Design review of the part built by this model. Coordinates are the model's own, in mm. Face numbers are marked on the shaded views. Coordinates: 2 decimals unless noted, no trailing zeros. Write each loop counter-clockwise with the first axis right and the second up, starting at its lowest first coordinate (ties: lowest second). Pieces come first, ordered by that corner, then holes. Notation, with made-up numbers: (20, -9.75) -> (49, -9.75) arc R23 cw to (49, 10.25) -> close; hole circle Ø11 at (78.25, -19.5). An arc over 180 degrees is marked (long way). Return JSON: item names as keys, results as strings. Group by question number.
Autodesk Inventor part; units mm, degrees
ref_plane "YZ Plane" through (0, 0, 0) normal (1, 0, 0) x (0, 1, 0)
ref_plane "XZ Plane" through (0, 0, 0) normal (0, 1, 0) x (-1, 0, 0)
ref_plane "XY Plane" through (0, 0, 0) normal (0, 0, 1) x (1, 0, 0)
sketch "Sketch1" plane through (0, 0, 0) normal (0, 1, 0) x (-1, 0, 0)
  line L0 (-34.1, -49) -> (34.1, -49)
  line L1 (34.1, -49) -> (34.1, 49)
  line L2 (34.1, 49) -> (-34.1, 49)
  line L3 (-34.1, 49) -> (-34.1, -49)
  line L4 (-34.1, -49) -> (34.1, 49) construction
  line L5 (34.1, -49) -> (-34.1, 49) construction
  circle A0 centre (-16.9, 39.55) radius 2
  circle A1 centre (-16.9, 39.55) radius 3.25
  line L6 (-18.8909, 27.1453) -> (-18.8909, 26.9568)
  circle A2 centre (-10.1, -20) radius 2
  circle A3 centre (-10.1, -20) radius 3.25
  point P0 (0, 0)
  dimension "d0" = 68.2
  dimension "d1" = 98
  dimension "d6" = 4
  dimension "d7" = 6.5
  dimension "d8" = 17.2
  dimension "d9" = 9.45
  dimension "d10" = 24
  dimension "d11" = 29
  dimension "d12" = 4
  dimension "d13" = 6.5
extrude "Extrusion1" add sketch "Sketch1" along normal blind 31.8 contours L3 L2 L1 L0 | A0 | A1 | A2 | A3
shell "Shell1" thickness 1.5 removed faces 1 at (11.3667, 31.8, 16.3333)
extrude "Extrusion2" add sketch "Sketch1" along normal blind 4.5 contours A1 | A3
sketch "Sketch2" plane through (-34.1, 0, 49) normal (0, 0, 1) x (1, 0, 0)
  line L0 (0, 0) -> (68.2, 0)
  line L1 (68.2, 0) -> (68.2, 31.8)
  line L2 (68.2, 0) -> (68.2, 31.8)
  line L3 (68.2, 1.5) -> (40, 1.5)
  line L4 (68, 6) -> (36, 6)
  line L5 (36, 6) -> (36, 4.5)
  line L6 (36, 4.5) -> (68, 4.5)
  line L7 (68, 4.5) -> (68, 6)
  line L8 (47.2, 17.65) -> (54.7, 17.65)
  line L9 (54.7, 17.65) -> (54.7, 14.9)
  line L10 (54.7, 14.9) -> (47.2, 14.9)
  line L11 (47.2, 14.9) -> (47.2, 17.65)
  line L12 (47.2, 17.65) -> (54.7, 14.9)
  line L13 (54.7, 17.65) -> (47.2, 14.9)
  line L14 (55.7, 13.9) -> (46.2, 13.9)
  line L15 (46.2, 13.9) -> (46.2, 18.65)
  line L16 (46.2, 18.65) -> (55.7, 18.65)
  line L17 (55.7, 18.65) -> (55.7, 13.9)
  line L18 (55.7, 13.9) -> (46.2, 18.65) construction
  line L19 (46.2, 13.9) -> (55.7, 18.65) construction
  point P0 (34.1, 0)
  point P1 (50.95, 16.275)
  dimension "d19" = 1.5
  dimension "d20" = 3
  dimension "d21" = 1.5
  dimension "d22" = 8.9
  dimension "d23" = 7.5
  dimension "d24" = 2.75
  dimension "d25" = 13.5
  dimension "d26" = 1
  dimension "d27" = 1
extrude "Extrusion3" cut sketch "Sketch2" against normal blind 4.5 contours L12 L13 L11 | L8 L13 L12 | L9 L12 L13 | L13 L12 L10 | L14 L15 L16 L17
fillet "Fillet1" radius 1 4 edges at (16.85, 18.65, 49) (21.6, 16.275, 49) (16.85, 13.9, 49) (12.1, 16.275, 49)
sketch "Sketch3" plane through (34.1, 0, 49) normal (1, 0, 0) x (0, 0, -1)
  line L0 (0, 0) -> (98, 0)
  line L1 (98, 0) -> (98, 31.8)
  line L2 (80.7, 17.4) -> (93.6, 17.4)
  line L3 (93.6, 17.4) -> (93.6, 6)
  line L4 (93.6, 6) -> (80.7, 6)
  line L5 (80.7, 6) -> (80.7, 17.4)
  line L6 (80.7, 17.4) -> (93.6, 6) construction
  line L7 (93.6, 17.4) -> (80.7, 6) construction
  line L8 (94.6, 5) -> (79.7, 5)
  line L9 (79.7, 5) -> (79.7, 18.4)
  line L10 (79.7, 18.4) -> (94.6, 18.4)
  line L11 (94.6, 18.4) -> (94.6, 5)
  line L12 (94.6, 5) -> (79.7, 18.4) construction
  line L13 (79.7, 5) -> (94.6, 18.4) construction
  point P0 (49, 0)
  point P1 (87.15, 11.7)
  point P2 (87.15, 11.7)
  dimension "d31" = 6
  dimension "d32" = 4.4
  dimension "d33" = 11.4
  dimension "d34" = 12.9
  dimension "d35" = 1
  dimension "d36" = 1
extrude "Extrusion4" cut sketch "Sketch3" against normal blind 4.5 contours L2 L3 L4 L5 | L8 L9 L10 L11
sketch "Sketch4" plane through (34.1, 0, -49) normal (0, 0, -1) x (-1, 0, 0)
  line L0 (0, 0) -> (68.2, 0)
  line L1 (0, 0) -> (0, 31.8)
  line L2 (28.8, 6) -> (20.1, 6)
  line L3 (20.1, 6) -> (20.1, 16.6)
  line L4 (20.1, 16.6) -> (28.8, 16.6)
  line L5 (28.8, 16.6) -> (28.8, 6)
  line L6 (28.8, 6) -> (20.1, 16.6) construction
  line L7 (20.1, 6) -> (28.8, 16.6) construction
  line L8 (29.8, 5) -> (19.1, 5)
  line L9 (19.1, 5) -> (19.1, 17.6)
  line L10 (19.1, 17.6) -> (29.8, 17.6)
  line L11 (29.8, 17.6) -> (29.8, 5)
  line L12 (29.8, 5) -> (19.1, 17.6) construction
  line L13 (19.1, 5) -> (29.8, 17.6) construction
  point P0 (34.1, 0)
  point P1 (24.45, 11.3)
  dimension "d39" = 20.1
  dimension "d40" = 6
  dimension "d41" = 8.7
  dimension "d42" = 10.6
  dimension "d43" = 1
  dimension "d44" = 1
extrude "Extrusion5" cut sketch "Sketch4" against normal blind 4.5 contours L2 L3 L4 L5 | L8 L9 L10 L11
sketch "Sketch5" plane through (0, 31.8, 0) normal (0, 1, 0) x (1, 0, 0)
  line L0 (32.6, -47.5) -> (-32.6, -47.5)
  line L1 (-32.6, -47.5) -> (-32.6, 47.5)
  line L2 (-32.6, 47.5) -> (32.6, 47.5)
  line L3 (32.6, 47.5) -> (32.6, -47.5)
  line L4 (34.1, -49) -> (34.1, 49)
  line L5 (34.1, 49) -> (-34.1, 49)
  line L6 (-34.1, 49) -> (-34.1, -49)
  line L7 (-34.1, -49) -> (34.1, -49)
  line L8 (34.1, -49) -> (-34.1, -49)
  line L9 (-34.1, -49) -> (-34.1, 49)
  line L10 (-34.1, 49) -> (34.1, 49)
  line L11 (34.1, 49) -> (34.1, -49)
  circle A0 centre (-23.6, -34.15) radius 3
  circle A1 centre (-23.6, -34.15) radius 3.5
  circle A2 centre (-5.6, -34.15) radius 3.5
  circle A3 centre (-23.6, -16.15) radius 3.5
  circle A4 centre (-5.6, -16.15) radius 3.5
  circle A5 centre (-23.6, 1.85) radius 3.5
  circle A6 centre (-5.6, 1.85) radius 3.5
  circle A7 centre (-23.6, 19.85) radius 3.5
  circle A8 centre (-5.6, 19.85) radius 3.5
  circle A9 centre (-23.6, 37.85) radius 3.5
  circle A10 centre (-5.6, 37.85) radius 3.5
  circle A11 centre (-5.6, 1.85) radius 3.5
  circle A12 centre (21.9, 19.85) radius 3.5
  circle A13 centre (21.9, 1.85) radius 3.5
  line L12 (34.1, -49) -> (-34.1, -49)
  line L13 (-34.1, -49) -> (-34.1, 49)
  line L14 (-34.1, 49) -> (34.1, 49)
  line L15 (34.1, 49) -> (34.1, -49)
  point P0 (0, 0)
  dimension "d47" = 6
  dimension "d48" = 7
  dimension "d50" = 13.35
  dimension "d51" = 9
  dimension "d54" = 18
  dimension "d57" = 18
  dimension "d62" = 18
  dimension "d65" = 18
  dimension "d70" = 18
  dimension "d73" = 27.5
extrude "Extrusion6" add sketch "Sketch5" along normal blind 1.5 contours L0 L1 L2 L3 | L7 L6 L5 L4
fillet "Fillet2" radius 2 4 edges at (34.1, 16.65, -49) (-34.1, 16.65, -49) (34.1, 16.65, 49) (-34.1, 16.65, 49)
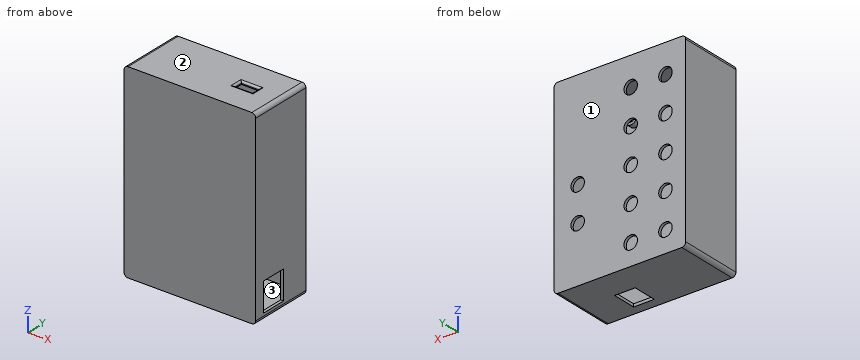
Q1. The part is to be moulded in two halves that separate along Y. For the marked faces 1, 2 and 3, say which applies: +Y half, -Y half, draft (parallel to the pull), parting line (faces both ways), or undercut.
Q2. We need section A-A on y = 30.5. Write out the cut boundary in (x, z).
Q3. Wall thickness on L1, parallel to Z at x = -23.6, y = 32.25; L2, parallel to X at y = 2.1, z = -20; L3, parallel to X at y = 24, z = -3.5: over which ranges is each line inside the solid? List them lowest first.
Q4. We need section C-C on z = 34.15. Write out the cut boundary in (x, y).
Q5. We need section B-B on x = -23.6. Write out the cut boundary in (y, z), plus the area to 3 significant figures.
Q6. For P1, Ø2, axis at x = 12, y = 13, coming from the -Z side; P2, Ø5.5, axis at x = -23.6, z = 16.15, coming from the +Y side, all flat-tipped, find the tip position at first contact; note any pin that passes through.
Q7. We need section D-D on y = 11.5. Write out the cut boundary in (x, z).
Findings below:
{
 "1": {"face 1": "+Y half", "face 2": "draft", "face 3": "undercut"},
 "2": {"outline": "(-34.1, -47) arc R2 ccw to (-32.1, -49) -> (32.1, -49) arc R2 ccw to (34.1, -47) -> (34.1, 47) arc R2 ccw to (32.1, 49) -> (-32.1, 49) arc R2 ccw to (-34.1, 47) -> close; hole (-32.6, -47.5) -> (32.6, -47.5) -> (32.6, 47.5) -> (-32.6, 47.5) -> close"},
 "3": {"L1": "z = -49 to -41.35, -34.35 to -23.35, -16.35 to -5.35, 1.65 to 12.65, 19.65 to 30.65, 37.65 to 49", "L2": "x = -34.1 to -32.6, 6.85 to 8.1, 12.1 to 13.35, 32.6 to 34.1", "L3": "x = -34.1 to -32.6, 32.6 to 34.1"},
 "4": {"outline": "(-34.1, 0) -> (34.1, 0) -> (34.1, 33.3) -> (-2.1, 33.3) -> (-2.1, 31.8) -> (32.6, 31.8) -> (32.6, 1.5) -> (-32.6, 1.5) -> (-32.6, 31.8) -> (-27.1, 31.8) -> (-27.1, 33.3) -> (-34.1, 33.3) -> close; (-20.1, 31.8) -> (-9.1, 31.8) -> (-9.1, 33.3) -> (-20.1, 33.3) -> close"},
 "5": {"outline": "(0, -49) -> (33.3, -49) -> (33.3, -41.35) -> (31.8, -41.35) -> (31.8, -47.5) -> (1.5, -47.5) -> (1.5, 47.5) -> (31.8, 47.5) -> (31.8, 37.65) -> (33.3, 37.65) -> (33.3, 49) -> (0, 49) -> close; (31.8, -34.35) -> (33.3, -34.35) -> (33.3, -23.35) -> (31.8, -23.35) -> close; (31.8, -16.35) -> (33.3, -16.35) -> (33.3, -5.35) -> (31.8, -5.35) -> close; (31.8, 1.65) -> (33.3, 1.65) -> (33.3, 12.65) -> (31.8, 12.65) -> close; (31.8, 19.65) -> (33.3, 19.65) -> (33.3, 30.65) -> (31.8, 30.65) -> close", "area": "332 mm^2"},
 "6": {"P1": "stops at z = 47.5", "P2": "stops at y = 1.5"},
 "7": {"outline": "(-34.1, -47) arc R2 ccw to (-32.1, -49) -> (4.3, -49) -> (4.3, -47.5) -> (-32.6, -47.5) -> (-32.6, 47.5) -> (32.6, 47.5) -> (32.6, -30.7) -> (34.1, -30.7) -> (34.1, 47) arc R2 ccw to (32.1, 49) -> (-32.1, 49) arc R2 ccw to (-34.1, 47) -> close; (15, -49) -> (32.1, -49) arc R2 ccw to (34.1, -47) -> (34.1, -45.6) -> (32.6, -45.6) -> (32.6, -47.5) -> (15, -47.5) -> close"}
}
